from build123d import *

# Parameters (mm, degrees)
SKETCH1_R                 = 22.5
BOSS_EXTRUDE1_DEPTH       = 20
CUT_EXTRUDE1_REACH        = 22
SKETCH3_R                 = 5
F_3_0MM_DOWEL_HOLE1_D     = 3
F_3_0MM_DOWEL_HOLE1_DEPTH = 22
F_3_0MM_DOWEL_HOLE1_TIP   = 0.901291
BOSS_EXTRUDE3_DEPTH       = 10


with BuildPart() as part:
    # Sketch1 → Boss-Extrude1 (new body)
    with BuildSketch(Plane.XY):
        Circle(SKETCH1_R)
    extrude(amount=BOSS_EXTRUDE1_DEPTH)

    # Sketch3 → Cut-Extrude1 (cut, up to next)
    with BuildSketch(Plane.XY.offset(20), mode=Mode.PRIVATE) as cut_extrude1_sk1:
        Circle(SKETCH3_R)
    cut_extrude1_tool1 = extrude(cut_extrude1_sk1.sketch, amount=-CUT_EXTRUDE1_REACH, mode=Mode.PRIVATE) & part.part
    add(cut_extrude1_tool1.solids().sort_by_distance((0, 0, 20))[0], mode=Mode.SUBTRACT)

    # Ø3.0mm Dowel Hole1
    with Locations(Plane(origin=(0.332625, 22.497541, 9.950984), x_dir=(0.999891, -0.014783, 0), z_dir=(0.014783, 0.999891, 0))):
        with Locations((0, 0)):
            Hole(F_3_0MM_DOWEL_HOLE1_D / 2, depth=F_3_0MM_DOWEL_HOLE1_DEPTH)
            with Locations((0, 0, -(F_3_0MM_DOWEL_HOLE1_DEPTH + F_3_0MM_DOWEL_HOLE1_TIP / 2))):  # 118° drill point
                Cone(0, F_3_0MM_DOWEL_HOLE1_D / 2, F_3_0MM_DOWEL_HOLE1_TIP, mode=Mode.SUBTRACT)

    # Sketch6 → Boss-Extrude3 (add)
    with BuildSketch(Plane.XY.offset(20)):
        with BuildLine():
            Line((-17.498377, 14.144144), (-10.881805, 10.324065))
            ThreePointArc((-10.881805, 10.324065), (-7.5, 12.990381), (-3.5, 14.585952))
            Line((-3.5, 14.585952), (-3.5, 22.226111))
            ThreePointArc((-3.5, 22.226111), (-11.25, 19.485572), (-17.498377, 14.144144))
        make_face()
        with BuildLine():
            Line((14.381805, 4.261887), (20.998377, 8.081966))
            ThreePointArc((20.998377, 8.081966), (22.5, 0), (20.998377, -8.081966))
            Line((20.998377, -8.081966), (14.381805, -4.261887))
            ThreePointArc((14.381805, -4.261887), (15, 0), (14.381805, 4.261887))
        make_face()
        with BuildLine():
            Line((-3.5, -14.585952), (-3.5, -22.226111))
            ThreePointArc((-3.5, -22.226111), (-11.25, -19.485572), (-17.498377, -14.144144))
            Line((-17.498377, -14.144144), (-10.881805, -10.324065))
            ThreePointArc((-10.881805, -10.324065), (-7.5, -12.990381), (-3.5, -14.585952))
        make_face()
    extrude(amount=BOSS_EXTRUDE3_DEPTH)


solid = part.part
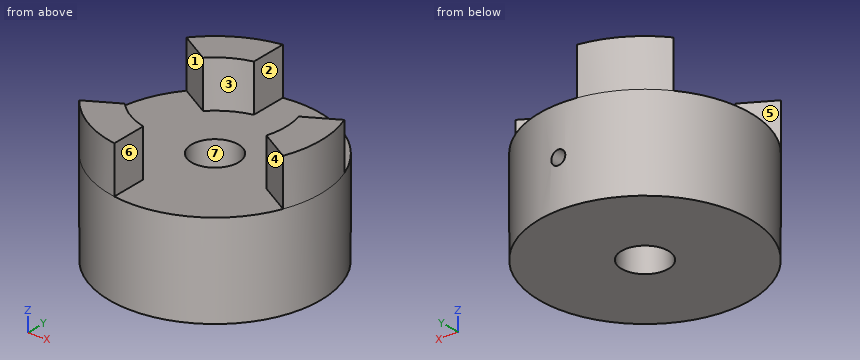
For this review, take the finished solid that the model builds, in its own axes (mm). Face numbers are marked on the shaded views. A direction names the side the tool comes from. Round coordinates to 2 decimals unless told otherwise and drop trailing zeros. Write each loop counter-clockwise with the first axis right and the second up, starting at its lowest first coordinate (ties: lowest second). Pieces come first, ordered by that corner, then holes. Notation, with made-up numbers: (-10, -20.75) - (10, -20.75) arc R13 ccw to (10, 0.25) - close; hole circle Ø7 at (-35.75, 55.5). An arc over 180 degrees is marked (long way). Write item = value, one per line. Start each with the question number.
1. Consider section C-C on x = -2. State the section outline as (y, z) points.
2. Consider section A-A on z = 28.5. State the section outline as (x, y) points, plus the area to 3 significant figures.
3. Consider section B-B on y = 0. State the section outline as (x, z) points.
4. Consider section D-D on y = -18. State the section outline as (x, z) points.
5. Wall thickness on L1, parallel to Y at x = 0, z = 8; L2, parallel to Z at x = 12, y = -7; L3, parallel to X at y = 0, z = 22: over which ranges is each line inside the solid? List them lowest first.
6. For the marked faces 1, 2 and 3, list the 3-axis set-ups (+Z, -Z, +X, -X, +Y, -Y) from which the entire face can be reached by the end or side of a thin tool; tool diameter is ignored.
7. For pin 1 Ø2.5 at (y, z) = (18, 24) entering from +X; pin 2 Ø2 at (x, z) = (14, 26) entering from +Y; pin 3 Ø2 at (x, y) = (4, -10.5) entering from +Z, all flat-tipped, find the tip position at first contact; note any pin that passes through.
8. Draft analysis for pull direction Y (two halves, no side actions). For the marked faces 4, 5, 6 and 7, state which applies: released by +Y, released by -Y, zero draft, split by the parting line, or undercut.
Evaluation:
q1.outline = (-22.41, 0) - (-4.58, 0) - (-4.58, 20) - (-22.41, 20) - close; (4.58, 0) - (22.41, 0) - (22.41, 20) - (4.58, 20) - close
q2.outline = (-17.5, -14.14) arc R22.5 ccw to (-3.5, -22.23) - (-3.5, -14.59) arc R15 cw to (-10.88, -10.32) - close; (-17.5, 14.14) - (-10.88, 10.32) arc R15 cw to (-3.5, 14.59) - (-3.5, 22.23) arc R22.5 ccw to start; (14.38, -4.26) - (21, -8.08) arc R22.5 ccw to (21, 8.08) - (14.38, 4.26) arc R15 cw to start
q2.area = 283 mm2
q3.outline = (-22.5, 0) - (-5, 0) - (-5, 20) - (-22.5, 20) - close; (5, 0) - (22.5, 0) - (22.5, 30) - (15, 30) - (15, 20) - (5, 20) - close
q4.outline = (-13.5, 0) - (13.5, 0) - (13.5, 20) - (-3.5, 20) - (-3.5, 30) - (-13.5, 30) - close
q5.L1 = -22.5 to -5, 5 to 22.5
q5.L2 = 0 to 20
q5.L3 = 15 to 22.5
q6.face_1 = +Z, -X
q6.face_2 = +Z, +X, +Y, -Y
q6.face_3 = +Z, +X
q7.pin_1 = -3.5
q7.pin_2 = 4.62
q7.pin_3 = 20
q8.face_4 = released by -Y
q8.face_5 = undercut
q8.face_6 = zero draft
q8.face_7 = undercut
